```python
from build123d import *

# Parameters (mm, degrees)
BOSS_EXTRUDE1_DEPTH = 6.35
SKETCH3_W           = 19.05
SKETCH3_H           = 38.1
CUT_EXTRUDE1_DEPTH  = 294.064711284


with BuildPart() as part:
    # Sketch1 → Boss-Extrude1 (new body)
    with BuildSketch(Plane(origin=(0, 0, 0), x_dir=(1, 0, 0), z_dir=(0, 1, 0))):
        with BuildLine():
            Line((3.81, 0), (250.19, 0))
            ThreePointArc((250.19, 0), (252.884076836, 1.115923164), (254, 3.81))
            Line((254, 3.81), (254, 142.24))
            ThreePointArc((254, 142.24), (252.884076836, 144.934076836), (250.19, 146.05))
            Line((250.19, 146.05), (3.81, 146.05))
            ThreePointArc((3.81, 146.05), (1.115923164, 144.934076836), (0, 142.24))
            Line((0, 142.24), (0, 3.81))
            ThreePointArc((0, 3.81), (1.115923164, 1.115923164), (3.81, 0))
        make_face()
        with BuildLine():
            Line((35.56, 142.025), (218.44, 142.025))
            ThreePointArc((218.44, 142.025), (221.134076836, 140.909076836), (222.25, 138.215))
            Line((222.25, 138.215), (222.25, 7.835))
            ThreePointArc((222.25, 7.835), (221.134076836, 5.140923164), (218.44, 4.025))
            Line((218.44, 4.025), (35.56, 4.025))
            ThreePointArc((35.56, 4.025), (32.865923164, 5.140923164), (31.75, 7.835))
            Line((31.75, 7.835), (31.75, 138.215))
            ThreePointArc((31.75, 138.215), (32.865923164, 140.909076836), (35.56, 142.025))
        make_face(mode=Mode.SUBTRACT)
    extrude(amount=BOSS_EXTRUDE1_DEPTH)

    # Sketch3 → Cut-Extrude1 (cut, through all)
    with BuildSketch(Plane.XZ):
        with Locations((231.775, -51.7525)):
            Rectangle(SKETCH3_W, SKETCH3_H)
        with Locations((22.225, -51.1175)):
            Rectangle(SKETCH3_W, SKETCH3_H)
    extrude(amount=-CUT_EXTRUDE1_DEPTH, mode=Mode.SUBTRACT)


solid = part.part
```
Can you work these out from the model? Positions are in its coordinate system, mm. A direction names the side the tool comes from. Give positions to 0.01 mm unless a question says otherwise; leave off trailing zeros. Write each loop counter-clockwise with the first axis right and the second up, starting at its lowest first coordinate (ties: lowest second). Pieces come first, ordered by that corner, then holes. Notation, with made-up numbers: (38, 61) - (76, 61) arc R23 cw to (76, 84) - close; hole circle Ø10 at (59, 13.25). An arc over 180 degrees is marked (long way). Write item = value, one per line. Start each with the question number.
1. On a 3-axis mill with a long thin cutter (end or side, diameter ignored), from which of +Z, -Z, +X, -X, +Y, -Y can I reach the whole of each face in a straight line? I mean faces 5 (the face through (254, 3, -72)), 6 (the face through (31.75, 3, -104)). Say none if no direction works.
2. Thinking about a two-plate mould opening in Z: for faces 1 (the face through (129, 3, -146.05)), 2 (the face through (125, 3, 0)), 3 (the face through (222.25, 3, -105)), 4 (the face through (126, 6.35, -144)), which applies, released by +Z, released by -Z, zero draft, split by the parting line, or undercut?
3. Imagine slicing it at A-A (x = 76.5). Please give me the cut outline in (y, z) (3 decimals).
4. Imagine slicing it at B-B (z = -108). Please give me the cut outline in (x, y), and give its area (3 significant figures).
5. Please list where these lines run through material, in increasing order: line 1 (X direction, y = 3, z = -34.5); line 2 (X direction, y = 5.25, z = -85.5); line 3 (Z direction, x = 202, y = 2) (3 decimals).
Worked answers:
q1.face_5 = +Z, -Z, +X, +Y, -Y
q1.face_6 = +Y, -Y
q2.face_1 = released by -Z
q2.face_2 = released by +Z
q2.face_3 = undercut
q2.face_4 = zero draft
q3.outline = (0, -146.05) - (6.35, -146.05) - (6.35, -142.025) - (0, -142.025) - close; (0, -4.025) - (6.35, -4.025) - (6.35, 0) - (0, 0) - close
q4.outline = (0, 0) - (31.75, 0) - (31.75, 6.35) - (0, 6.35) - close; (222.25, 0) - (254, 0) - (254, 6.35) - (222.25, 6.35) - close
q4.area = 403 mm2
q5.line_1 = 0 to 12.7, 241.3 to 254
q5.line_2 = 0 to 31.75, 222.25 to 254
q5.line_3 = -146.05 to -142.025, -4.025 to 0
